The listing builds one solid part. Answer for the finished solid, in the listing's coordinates (mm). A direction names the side the tool comes from. Coordinates: 2 decimals unless noted, no trailing zeros. Loops run counter-clockwise (first coordinate to the right, second up) from the corner with the lowest first, then second, coordinate; pieces in that order, holes last. Notation, with made-up numbers: (64, 14.5) - (80, 14.5) arc R5 ccw to (80, 20.5) - close; hole circle Ø2 at (84, -4). An arc over 180 degrees is marked (long way). Return JSON: item names as keys, results as strings. Group by question number.
1. Section D-D (x = 368) is taken. Write down the section's boundary in (y, z) (3 decimals), and give its area (3 significant figures).
2. Section A-A (x = -10) is taken. Write down the section's boundary in (y, z) (1 decimal), and give its area (3 significant figures).
3. Which of the six approach directions +Z, -Z, +X, -X, +Y, -Y give full straight-line access (tool end or side, diameter ignored) to faces 1 (the face through (97, -408, 0)), 2 (the face through (-149.264, -386.181, 1.61))?
4. Section B-B (y = -148) is taken. Write down the section's boundary in (x, z) (3 decimals), and give its area (3 significant figures).
5. Find the intervals of material crossed by line 1 along Y through (x, z) = (133, 2.45); line 2 along X through (y, z) = (-246, 1.45); line 3 along Y through (x, z) = (-104.5, 2.65), in increasing order.
6. The mould has two halves that part along Y. Classify faces 3 (the face through (97, -408, 3.175)), 4 (the face through (-72.158, -226.581, 1.61)), 5 (the face through (-47, -81.41, 1.57)): pulls with the +Y half, pulls with the -Y half, needs draft (parallel to the pull), parting line crosses it, or undercut.
7. Section C-C (y = -421) is taken. Write down the section's boundary in (x, z) (3 decimals).
8. Each of these flat-tipped pins is pushed along its axis until it touches: P1, Ø1.5, axis at x = -30.5, z = 2.5, coming from the +Y side; P2, Ø1, axis at y = -450, z = 1, coming from the +X side; P3, Ø1.6, axis at y = -449.5, z = 2, coming from the +X side. Where does it stop, or does it pass through?
```python
from build123d import *

# Parameters (mm, degrees)
BOSS_EXTRUDE1_DEPTH = 3.175
SKETCH2_W           = 12.7
SKETCH2_H           = 25.4
CUT_EXTRUDE1_DEPTH  = 612.325617511
SKETCH4_W           = 88.9
SKETCH4_H           = 3.175
CUT_EXTRUDE2_DEPTH  = 612.325617511
CUT_EXTRUDE3_DEPTH  = 612.325617511
CUT_EXTRUDE4_DEPTH  = 612.325617511


with BuildPart() as part:
    # Sketch1 → Boss-Extrude1 (new body)
    with BuildSketch(Plane.XY):
        Polygon((0, 0), (190.5, 0), (412.75, -384.948291982), (374.65, -450.939427751), (-184.15, -450.939427751), (-222.25, -384.948291982), align=None)
    extrude(amount=BOSS_EXTRUDE1_DEPTH)

    # Sketch2 → Cut-Extrude1 (cut, through all)
    with BuildSketch(Plane.XY.offset(3.175)):
        with Locations((69.85, -12.7)):
            Rectangle(SKETCH2_W, SKETCH2_H)
        with BuildLine():
            Line((29.329393675, -76.2), (161.170606325, -76.2))
            ThreePointArc((161.170606325, -76.2), (173.870606325, -79.602954744), (183.167651581, -88.9))
            Line((183.167651581, -88.9), (339.952954744, -360.460110958))
            ThreePointArc((339.952954744, -360.460110958), (339.952954744, -385.860110958), (317.955909488, -398.560110958))
            Line((317.955909488, -398.560110958), (-127.455909488, -398.560110958))
            ThreePointArc((-127.455909488, -398.560110958), (-149.452954744, -385.860110958), (-149.452954744, -360.460110958))
            Line((-149.452954744, -360.460110958), (7.332348419, -88.9))
            ThreePointArc((7.332348419, -88.9), (16.629393675, -79.602954744), (29.329393675, -76.2))
        make_face()
        with Locations((120.65, -12.7)):
            Rectangle(SKETCH2_W, SKETCH2_H)
    extrude(amount=-CUT_EXTRUDE1_DEPTH, mode=Mode.SUBTRACT)

    # Sketch4 → Cut-Extrude2 (cut, through all)
    with BuildSketch(Plane.XY.offset(3.175)):
        with Locations((-114.3, -449.351927751)):
            Rectangle(SKETCH4_W, SKETCH4_H)
        with Locations((25.4, -449.351927751)):
            Rectangle(SKETCH4_W, SKETCH4_H)
        with Locations((165.1, -449.351927751)):
            Rectangle(SKETCH4_W, SKETCH4_H)
        with Locations((304.8, -449.351927751)):
            Rectangle(SKETCH4_W, SKETCH4_H)
        Polygon((-215.9, -395.94681461), (-214.525184671, -395.15306461), (-189.125184671, -439.147155122), (-190.5, -439.940905122), align=None)
        Polygon((406.4, -395.94681461), (405.025184671, -395.15306461), (379.625184671, -439.147155122), (381, -439.940905122), align=None)
    extrude(amount=-CUT_EXTRUDE2_DEPTH, mode=Mode.SUBTRACT)

    # Sketch5 → Cut-Extrude3 (cut, through all)
    with BuildSketch(Plane.XY.offset(3.175)):
        Polygon((-208.788, -361.631424011), (-207.413184671, -362.425174011), (-168.424184671, -294.894245074), (-169.799, -294.100495074), align=None)
        Polygon((-143.024184671, -250.900154562), (-104.035184671, -183.369225626), (-105.41, -182.575475626), (-144.399, -250.106404562), align=None)
        Polygon((399.288, -361.631424011), (397.913184671, -362.425174011), (358.924184671, -294.894245074), (360.299, -294.100495074), align=None)
        Polygon((334.899, -250.106404562), (333.524184671, -250.900154562), (294.535184671, -183.369225626), (295.91, -182.575475626), align=None)
    extrude(amount=-CUT_EXTRUDE3_DEPTH, mode=Mode.SUBTRACT)

    # Sketch6 → Cut-Extrude4 (cut, through all)
    with BuildSketch(Plane.XY.offset(3.175)):
        Polygon((-155.829, -269.903745293), (-148.954923357, -273.872495293), (-152.129923357, -279.371756607), (-159.004, -275.403006607), align=None)
        Polygon((349.504, -275.403006607), (346.329, -269.903745293), (339.454923357, -273.872495293), (342.629923357, -279.371756607), align=None)
        Polygon((-205.215923357, -371.319405777), (-208.390923357, -376.818667091), (-215.265, -372.849917091), (-212.09, -367.350655777), align=None)
        Polygon((-85.835923357, -164.54718037), (-89.010923357, -170.046441684), (-95.885, -166.077691684), (-92.71, -160.57843037), align=None)
        Polygon((286.385, -166.077691684), (283.21, -160.57843037), (276.335923357, -164.54718037), (279.510923357, -170.046441684), align=None)
        Polygon((405.765, -372.849917091), (402.59, -367.350655777), (395.715923357, -371.319405777), (398.890923357, -376.818667091), align=None)
    extrude(amount=-CUT_EXTRUDE4_DEPTH, mode=Mode.SUBTRACT)


solid = part.part
```
The answers:
{
 "1": {"outline": "(-450.939, 0) - (-310.614, 0) - (-310.614, 3.175) - (-450.939, 3.175) - close", "area": "446 mm2"},
 "2": {"outline": "(-447.8, 0) - (-398.6, 0) - (-398.6, 3.2) - (-447.8, 3.2) - close; (-118.9, 0) - (-17.3, 0) - (-17.3, 3.2) - (-118.9, 3.2) - close", "area": "479 mm2"},
 "3": {"face 1": "-Z, +X, -X, +Y, -Y", "face 2": "+Z, -Z"},
 "4": {"outline": "(-85.448, 0) - (-26.789, 0) - (-26.789, 3.175) - (-85.448, 3.175) - close; (217.289, 0) - (275.948, 0) - (275.948, 3.175) - (217.289, 3.175) - close", "area": "372 mm2"},
 "5": {"line 1": "y = -447.76 to -398.56, -76.2 to 0", "line 2": "x = -140.2 to -83.37, 273.87 to 330.7", "line 3": "y = -447.76 to -398.56, -282.6 to -184.17, -183.1 to -181"},
 "6": {"face 3": "needs draft", "face 4": "undercut", "face 5": "pulls with the +Y half"},
 "7": {"outline": "(-199.602, 0) - (390.102, 0) - (390.102, 3.175) - (-199.602, 3.175) - close"},
 "8": {"P1": "stops at y = -51.53", "P2": "stops at x = 375.48", "P3": "stops at x = 375.94"}
}
